```python
from build123d import *

# Parameters (mm, degrees)
SKETCH1_W           = 118
SKETCH1_H           = 168
BOSS_EXTRUDE1_DEPTH = 5
SKETCH2_W           = 118
SKETCH2_H           = 168
SKETCH2_W_2         = 110
SKETCH2_H_2         = 160
BOSS_EXTRUDE2_DEPTH = 60
SKETCH3_W           = 13
SKETCH3_H           = 14
SKETCH3_W_2         = 11
CUT_EXTRUDE1_DEPTH  = 10
SKETCH4_W           = 98
SKETCH4_H           = 50.5
CUT_EXTRUDE2_DEPTH  = 2
CUT_EXTRUDE3_DEPTH  = 10
SKETCH6_W           = 3
SKETCH6_H           = 17
BOSS_EXTRUDE3_DEPTH = 12
REVOLVE2_ANGLE      = 180
FILLET1_R           = 5
SKETCH10_W          = 110
SKETCH10_H          = 5
CUT_EXTRUDE4_DEPTH  = 12
SKETCH11_W          = 2
SKETCH11_H          = 2
BOSS_EXTRUDE4_DEPTH = 160


with BuildPart() as part:
    # Sketch1 → Boss-Extrude1 (new body)
    with BuildSketch(Plane(origin=(0, 0, 0), x_dir=(1, 0, 0), z_dir=(0, 1, 0))):
        with Locations((59, 84)):
            Rectangle(SKETCH1_W, SKETCH1_H)
    extrude(amount=BOSS_EXTRUDE1_DEPTH)

    # Sketch2 → Boss-Extrude2 (add)
    with BuildSketch(Plane(origin=(0, 5, 0), x_dir=(1, 0, 0), z_dir=(0, 1, 0))):
        with Locations((59, 84)):
            Rectangle(SKETCH2_W, SKETCH2_H)
        with Locations((59, 84)):
            Rectangle(SKETCH2_W_2, SKETCH2_H_2, mode=Mode.SUBTRACT)
    extrude(amount=BOSS_EXTRUDE2_DEPTH)

    # Sketch3 → Cut-Extrude1 (cut)
    with BuildSketch(Plane.ZY.offset(-114)):
        with Locations((-19, 12)):
            Rectangle(SKETCH3_W, SKETCH3_H)
        with Locations((-47, 12)):
            Rectangle(SKETCH3_W_2, SKETCH3_H)
    extrude(amount=-CUT_EXTRUDE1_DEPTH, mode=Mode.SUBTRACT)

    # Sketch4 → Cut-Extrude2 (cut)
    with BuildSketch(Plane(origin=(0, 5, 0), x_dir=(1, 0, 0), z_dir=(0, 1, 0))):
        with Locations((61, 31.75)):
            Rectangle(SKETCH4_W, SKETCH4_H)
    extrude(amount=-CUT_EXTRUDE2_DEPTH, mode=Mode.SUBTRACT)

    # Sketch5 → Cut-Extrude3 (cut)
    with BuildSketch(Plane.XY.offset(-164)):
        with BuildLine():
            Line((59, 5), (90, 5))
            Line((90, 5), (90, 25))
            ThreePointArc((90, 25), (84.369036145, 31.688760758), (76.5, 35.5))
            Line((76.5, 35.5), (41.5, 35.5))
            ThreePointArc((41.5, 35.5), (33.630963855, 31.688760758), (28, 25))
            Line((28, 25), (28, 5))
            Line((28, 5), (59, 5))
        make_face()
    extrude(amount=-CUT_EXTRUDE3_DEPTH, mode=Mode.SUBTRACT)

    # Sketch6 → Boss-Extrude3 (add)
    with BuildSketch(Plane.XY.offset(-164)):
        with Locations((26.5, 13.5)):
            Rectangle(SKETCH6_W, SKETCH6_H)
        with Locations((91.5, 13.5)):
            Rectangle(SKETCH6_W, SKETCH6_H)
    extrude(amount=BOSS_EXTRUDE3_DEPTH)

    # Sketch7 → Revolve1 (revolve)
    with BuildSketch(Plane(origin=(28, 0, 0), x_dir=(0, 0, -1), z_dir=(1, 0, 0))):
        with BuildLine():
            Line((157, 13), (163, 13))
            ThreePointArc((163, 13), (160, 10), (157, 13))
        make_face()
    revolve(axis=Axis((28, 13, -157), (0, 0, -1)))

    # Sketch9 → Revolve2 (revolve)
    with BuildSketch(Plane.ZY.offset(-90)):
        with BuildLine():
            Line((-163, 13), (-157, 13))
            ThreePointArc((-157, 13), (-160, 10), (-163, 13))
        make_face()
    revolve(axis=Axis((90, 13, -163), (0, 0, -1)), revolution_arc=REVOLVE2_ANGLE)

    # Fillet1
    fillet1_edges = [part.edges().sort_by_distance(p)[0] for p in [
        (91.5, 22, -152),
        (91.5, 22, -164),
        (26.5, 22, -164),
        (26.5, 22, -152),
    ]]
    fillet(fillet1_edges, radius=FILLET1_R)

    # Sketch10 → Cut-Extrude4 (cut)
    with BuildSketch(Plane(origin=(0, 0, -4), x_dir=(-1, 0, 0), z_dir=(0, 0, -1))):
        with Locations((-59, 62.5)):
            Rectangle(SKETCH10_W, SKETCH10_H)
    extrude(amount=-CUT_EXTRUDE4_DEPTH, mode=Mode.SUBTRACT)

    # Sketch11 → Boss-Extrude4 (add)
    with BuildSketch(Plane(origin=(0, 0, -4), x_dir=(-1, 0, 0), z_dir=(0, 0, -1))):
        Polygon((-114, 60), (-114, 58), (-112, 60), align=None)
        Polygon((-4, 60), (-4, 58), (-6, 60), align=None)
        with Locations((-113, 64)):
            Rectangle(SKETCH11_W, SKETCH11_H)
        with Locations((-5, 64)):
            Rectangle(SKETCH11_W, SKETCH11_H)
    extrude(amount=BOSS_EXTRUDE4_DEPTH)


solid = part.part
```
Model file for the job. Use its own axes, mm. A direction names the side the tool comes from. Coordinates: 2 decimals unless noted, no trailing zeros. Order: outer loops, then holes, each group sorted by start corner. A loop starts at its lowest first (then second) coordinate and runs counter-clockwise, first axis right, second up. Notation, with made-up numbers: (24.25, 12) - (41.25, 12) arc R26 cw to (41.25, 31) - close; hole circle Ø5 at (23, 45). An arc over 180 degrees is marked (long way). Return JSON: item names as keys, results as strings. Group by question number.
1) Saw through at A-A, the plane z = -21. Write the cut outline in (x, y).
2) Saw through at D-D, the plane x = 82.5. Write the cut outline in (y, z), plus the area to 3 significant figures.
3) Flat gauge pins, fed straight in: P1, Ø8, axis at x = 92, z = -84, coming from the +Y side; P2, Ø15, axis at x = 57.5, z = -43.5, coming from the +Y side; P3, Ø2, axis at x = 5.5, y = 64, coming from the +Z side. Where does each tip first touch, or does it go through?
4) Mould opens along X. For faces 1 (the flat face through (28, 17, -160)), 2 (the flat face through (59, 65, -165)), 3 (the flat face through (118, 32, -83)) say: released by +X, released by -X, zero draft, split by the parting line, or undercut.
5) Saw through at B-B, the plane y = 51.5. Write the cut outline in (x, z), plus the area to 3 significant figures.
6) Tool access for faces 4 (the flat face through (25, 13, -158)), 5 (the flat face through (116, 12, -52.5)), 6 (the flat face through (5.78, 60, -45.17)): list every direction of +Z, -Z, +X, -X, +Y, -Y with a clear straight run to the whole face (end or side of a thin tool).
7) Probe line 1 (Z direction, x = 71, y = 55.5); line 2 (X direction, y = 54, z = -105); line 3 (Z direction, x = 90.5, y = 24). List the from-to ranges inside material, lowest first. Write a range as from..to.
8) Saw through at C-C, the plane x = 19.5. Write the cut outline in (y, z).
Values found:
{
 "1": {"outline": "(0, 0) - (118, 0) - (118, 5) - (110, 5) - (110, 3) - (12, 3) - (12, 5) - (4, 5) - (4, 58) - (6, 60) - (4, 60) - (4, 63) - (6, 63) - (6, 65) - (0, 65) - close; (112, 60) - (114, 58) - (114, 19) - (118, 19) - (118, 65) - (112, 65) - (112, 63) - (114, 63) - (114, 60) - close"},
 "2": {"outline": "(0, -168) - (5, -168) - (5, -57) - (3, -57) - (3, -6.5) - (5, -6.5) - (5, -4) - (60, -4) - (60, 0) - (0, 0) - close; (32.99, -168) - (65, -168) - (65, -164) - (32.99, -164) - close", "area": "1,090 mm²"},
 "3": {"P1": "stops at y = 5", "P2": "stops at y = 3", "P3": "stops at z = -4"},
 "4": {"face 1": "undercut", "face 2": "zero draft", "face 3": "released by +X"},
 "5": {"outline": "(0, -168) - (118, -168) - (118, 0) - (0, 0) - close; hole (4, -164) - (114, -164) - (114, -4) - (4, -4) - close", "area": "2,220 mm²"},
 "6": {"face 4": "+Y", "face 5": "+X", "face 6": "+Z"},
 "7": {"line 1": "z = -168..-164, -4..0", "line 2": "x = 0..4, 114..118", "line 3": "z = -168..-163, -4..0"},
 "8": {"outline": "(0, -168) - (65, -168) - (65, -164) - (5, -164) - (5, -57) - (3, -57) - (3, -6.5) - (5, -6.5) - (5, -4) - (60, -4) - (60, 0) - (0, 0) - close"}
}
